Geometry check sheet. Reference: the model listing, model coordinates, mm. A direction names the side the tool comes from. Coordinates: 2 decimals unless noted, no trailing zeros. Write each loop counter-clockwise with the first axis right and the second up, starting at its lowest first coordinate (ties: lowest second). Pieces come first, ordered by that corner, then holes. Notation, with made-up numbers: (-2.5, -16) -> (34.5, -16) arc R14 ccw to (34.5, 7) -> close; hole circle Ø3 at (3, -8). An arc over 180 degrees is marked (long way). Answer in a Markdown table with one row per item. Add a question column.
Q1. Section check C-C, the plane y = 7.5. Record the boundary of the cut face in (x, z), and give its area (3 significant figures).
Q2. Tool access check on faces 1 (the face through (2, 5, -8)), 2 (the face through (13.55, -3.87, -14.5)), 3 (the face through (12.01, -0.73, -35.46)). Record the directions out of +Z, -Z, +X, -X, +Y, -Y that give a thin tool (end or side, any length) a straight path to the whole face; none if there is none.
Q3. Thickness scan on line 1 (Z direction, x = 12.7, y = -3.5); line 2 (X direction, y = -3.75, z = -38.56) (1 decimal); line 3 (X direction, y = -1.75, z = -23.5) (3 decimals). Record the ranges inside material, lowest first.
Q4. Release check for a two-part mould opening along Y. For faces 4 (the face through (9.754, 5.157, -1.521)), 5 (the face through (23, -2, -9.9)), 6 (the face through (41, 12.7, -1)) record: pulls with the +Y half, pulls with the -Y half, needs draft (parallel to the pull), parting line crosses it, or undercut.
Q5. Gauge pin test, flat ends, axial feed: P1, Ø7, axis at x = 33, z = -12, coming from the +Y side; P2, Ø2, axis at x = 16, y = -3.5, coming from the +Z side; P3, Ø1.9, axis at x = 13.5, z = -37.5, coming from the +Y side; P4, Ø5, axis at x = 36, y = 4, coming from the -Z side. Record the tip position at first contact, or that the pin passes through.
Q6. Section check B-B, the plane z = -13.16. Count the separate pieces of the cut face and the enclosed holes in it, and give its area (3 significant figures).
Q7. Section check D-D, the plane z = -21. Record the boundary of the cut face in (x, y) (3 decimals).
Q8. Section check A-A, the plane x = 8. Record the boundary of the cut face in (y, z), and give its area (3 significant figures).
Autodesk Inventor part; units mm, degrees
ref_plane "YZ Plane" through (0, 0, 0) normal (1, 0, 0) x (0, 1, 0)
ref_plane "XZ Plane" through (0, 0, 0) normal (0, 1, 0) x (-1, 0, 0)
ref_plane "XY Plane" through (0, 0, 0) normal (0, 0, 1) x (1, 0, 0)
sketch "Sketch1" plane through (0, 0, 0) normal (0, 0, 1) x (1, 0, 0)
  line L0 (0, 0) -> (47, 0)
  line L1 (47, 0) -> (47, 12.7)
  line L2 (47, 12.7) -> (0, 12.7)
  line L3 (0, 12.7) -> (0, 0)
  dimension "d0" = 47
  dimension "d1" = 12.7
extrude "Extrusion1" add sketch "Sketch1" against normal blind 3
sketch "Sketch2" plane through (0, 0, 0) normal (0, -1, 0) x (1, 0, 0)
  line L0 (47, 0) -> (0, 0)
  line L1 (0, 0) -> (0, -48)
  line L2 (0, -48) -> (47, -48)
  line L3 (47, -48) -> (47, 0)
  line L4 (47, 0) -> (47, -3)
  line L5 (47, 0) -> (0, 0)
  dimension "d6" = 0
  dimension "d24" = 48
  dimension "d25" = 0
extrude "Extrusion2" add sketch "Sketch2" along normal blind 5.2832
sketch "Sketch3" plane through (0, 0, -3) normal (0, 0, -1) x (-1, 0, 0)
  line L0 (-47, 12.7) -> (-47, 0)
  line L1 (-47, 0) -> (0, 0)
  line L2 (-47, 12.7) -> (-45, 12.7)
  line L3 (-45, 12.7) -> (-45, 0)
  line L4 (-45, 0) -> (-47, 0)
  line L5 (-47, 0) -> (-47, 12.7)
  line L6 (0, 0) -> (0, 12.7)
  line L7 (0, 0) -> (-2, 0)
  line L8 (-2, 0) -> (-2, 12.7)
  line L9 (-2, 12.7) -> (0, 12.7)
  line L10 (0, 12.7) -> (0, 0)
  dimension "d7" = 2
  dimension "d8" = 2
  dimension "d9" = 12.7
extrude "Extrusion3" add sketch "Sketch3" along normal blind 12.7
chamfer "Chamfer1" distance 12.7 angle 45 2 edges at (46, 12.7, -15.7) (1, 12.7, -15.7)
sketch "Sketch4" plane through (0, 0, -3) normal (0, 0, -1) x (-1, 0, 0)
  circle A0 centre (-39.0056, 5.08) radius 1.75
  circle A1 centre (-8.0056, 5.08) radius 1.75
  line L0 (-45, 0) -> (-45, 12.7)
  line L1 (-2, 12.7) -> (-2, 0)
  line L2 (0, 0) -> (-47, 0)
  dimension "d15" = 3.5
  dimension "d16" = 3.5
  dimension "d17" = 5.9944
  dimension "d18" = 31
  dimension "d19" = 6.0056
  dimension "d20" = 5.08
  dimension "d21" = 5.08
extrude "Extrusion4" cut sketch "Sketch4" against normal blind 12.7
sketch "Sketch5" plane through (0, 0, 0) normal (0, 0, 1) x (1, 0, 0)
  circle A0 centre (23.5, 15.7168) radius 12
  line L0 (47, -5.2832) -> (47, 12.7)
  line L1 (47, -5.2832) -> (0, -5.2832)
  point P0 (0, 0)
  dimension "d26" = 24
  dimension "d27" = 23.5
  dimension "d28" = 21
extrude "Extrusion5" cut sketch "Sketch5" against normal blind 5.2832
sketch "Sketch6" plane through (0, 0, 0) normal (0, 1, 0) x (1, 0, 0)
  circle A0 centre (12.7, 13.16) radius 1.5875
  circle A1 centre (12.7, 38.56) radius 1.5875
  circle A2 centre (34.3, 38.56) radius 1.5875
  circle A3 centre (34.3, 13.16) radius 1.5875
  line L0 (2, 3) -> (11.8854, 3)
  line L1 (0, 15.7) -> (0, 48)
  line L2 (47, 48) -> (47, 15.7)
  point P0 (0, 0)
  dimension "d31" = 3.175
  dimension "d32" = 3.175
  dimension "d33" = 3.175
  dimension "d34" = 3.175
  dimension "d35" = 10.16
  dimension "d36" = 25.4
  dimension "d37" = 25.4
  dimension "d38" = 10.16
  dimension "d39" = 12.7
  dimension "d40" = 12.7
  dimension "d41" = 12.7
  dimension "d42" = 12.7
extrude "Extrusion6" cut sketch "Sketch6" against normal blind 5.2832
sketch "Sketch7" plane through (0, 0, 0) normal (0, 1, 0) x (1, 0, 0)
  circle A0 centre (12.7, 13.16) radius 1.5875
  circle A1 centre (12.7, 13.16) radius 3.175
  circle A2 centre (12.7, 38.56) radius 1.5875
  circle A3 centre (12.7, 38.56) radius 3.175
  circle A4 centre (34.3, 13.16) radius 1.5875
  circle A5 centre (34.3, 13.16) radius 3.175
  circle A6 centre (34.3, 38.56) radius 1.5875
  circle A7 centre (34.3, 38.56) radius 3.175
  point P0 (0, 0)
  dimension "d45" = 6.35
  dimension "d46" = 6.35
  dimension "d47" = 6.35
  dimension "d48" = 6.35
extrude "Extrusion7" cut sketch "Sketch7" against normal blind 1.4732 contours A0 | A1 | A2 | A3 | A4 | A5 | A6 | A7
chamfer "Chamfer2" distance 1.016 angle 45 4 edges at (11.1125, -1.4732, -13.16) (32.7125, -1.4732, -13.16) (11.1125, -1.4732, -38.56) (32.7125, -1.4732, -38.56)
sketch "Sketch8" plane through (0, 0, 0) normal (0, 1, 0) x (1, 0, 0)
  line L0 (4.445, 20.06) -> (42.545, 20.06)
  line L1 (42.545, 20.06) -> (42.545, 32.76)
  line L2 (42.545, 32.76) -> (4.445, 32.76)
  line L3 (4.445, 32.76) -> (4.445, 20.06)
  line L4 (17.145, 9.9) -> (29.845, 9.9)
  line L5 (29.845, 9.9) -> (29.845, 41.65)
  line L6 (29.845, 41.65) -> (17.145, 41.65)
  line L7 (17.145, 41.65) -> (17.145, 9.9)
  line L8 (0, 15.7) -> (0, 48)
  line L9 (47, 48) -> (47, 15.7)
  line L10 (0, 48) -> (47, 48)
  point P0 (0, 0)
  point P1 (17.145, 20.06)
  point P2 (29.845, 20.06)
  point P3 (29.845, 32.76)
  point P4 (17.145, 32.76)
  dimension "d54" = 12.7
  dimension "d55" = 38.1
  dimension "d56" = 4.445
  dimension "d57" = 4.455
  dimension "d58" = 15.24
  dimension "d59" = 12.7
  dimension "d60" = 17.145
  dimension "d61" = 17.155
  dimension "d62" = 31.75
  dimension "d63" = 6.35
extrude "Extrusion8" cut sketch "Sketch8" against normal blind 3.81
chamfer "Chamfer3" distance 1.016 angle 45 12 edges at (10.795, 0, -20.06) (4.445, 0, -26.41) (10.795, 0, -32.76) (17.145, 0, -37.205) (23.495, 0, -41.65) (29.845, 0, -37.205) (36.195, 0, -32.76) (42.545, 0, -26.41) (36.195, 0, -20.06) (29.845, 0, -14.98) (23.495, 0, -9.9) (17.145, 0, -14.98)
properties part number "StepperMount"
Calculated:
| question | item | result |
|---|---|---|
| 1 | outline | (0, -8.2) -> (2, -8.2) -> (2, -3) -> (14.75, -3) -> (14.75, 0) -> (0, 0) -> close; (32.25, -3) -> (45, -3) -> (45, -8.2) -> (47, -8.2) -> (47, 0) -> (32.25, 0) -> close |
| 1 | area | 109 mm² |
| 2 | face 1 | -Z, +Y |
| 2 | face 2 | +Y, -Y |
| 2 | face 3 | +Y |
| 3 | line 1 | z = -48 to -40.15, -36.97 to -32.76, -20.06 to -14.75, -11.57 to 0 |
| 3 | line 2 | x = 0 to 11.1, 14.3 to 17.1, 29.8 to 32.7, 35.9 to 47 |
| 3 | line 3 | x = 0 to 4.445, 42.545 to 47 |
| 4 | face 4 | undercut |
| 4 | face 5 | needs draft |
| 4 | face 6 | pulls with the +Y half |
| 5 | P1 | stops at y = 0 |
| 5 | P2 | stops at z = 0 |
| 5 | P3 | stops at y = -1.8 |
| 5 | P4 | stops at z = -3 |
| 6 | separate pieces | 3 |
| 6 | enclosed holes | 0 |
| 6 | area | 164 mm² |
| 7 | outline | (0, -5.283) -> (47, -5.283) -> (47, 0) -> (43.561, 0) -> (42.545, -1.016) -> (42.545, -3.81) -> (4.445, -3.81) -> (4.445, -1.016) -> (3.429, 0) -> (0, 0) -> close |
| 8 | outline | (-5.28, -48) -> (0, -48) -> (0, -33.78) -> (-1.02, -32.76) -> (-3.81, -32.76) -> (-3.81, -20.06) -> (-1.02, -20.06) -> (0, -19.04) -> (0, -3) -> (3.33, -3) -> (3.33, 0) -> (-5.28, 0) -> close; (6.83, -3) -> (12.7, -3) -> (12.7, 0) -> (6.83, 0) -> close |
| 8 | area | 232 mm² |
